Autodesk Inventor part; units mm, degrees
ref_plane "YZ Plane" through (0, 0, 0) normal (1, 0, 0) x (0, 1, 0)
ref_plane "XZ Plane" through (0, 0, 0) normal (0, 1, 0) x (-1, 0, 0)
ref_plane "XY Plane" through (0, 0, 0) normal (0, 0, 1) x (1, 0, 0)
ref_plane "作業平面1" through (0, 0, 0) normal (0, 0, 1) x (1, 0, 0)
sketch "スケッチ1" plane through (0, 0, 0) normal (0, 0, 1) x (1, 0, 0)
  circle A0 centre (16.5, -9.9) radius 0.8
  circle A1 centre (-18.5, 9.9) radius 0.8
  circle A2 centre (16.5, 9.9) radius 0.8
  circle A3 centre (-18.5, -9.9) radius 0.8
  arc A4 (-21.5, -7.9) -> (-23.5, -9.9) centre (-21.5, -9.9) ccw
  line L0 (-23.5, -9.9) -> (-23.5, -11.9)
  line L1 (-23.5, -11.9) -> (23.5, -11.9)
  line L2 (23.5, -11.9) -> (23.5, 11.9)
  line L3 (23.5, 11.9) -> (-23.5, 11.9)
  line L4 (-23.5, 11.9) -> (-23.5, 9.9)
  arc A5 (-23.5, 9.9) -> (-21.5, 7.9) centre (-21.5, 9.9) ccw
  line L5 (-21.5, 7.9) -> (21.5, 7.9)
  line L6 (21.5, 7.9) -> (21.5, -7.9)
  line L7 (21.5, -7.9) -> (-21.5, -7.9)
  line L8 (-21.5, 11.9) -> (-21.5, -11.9)
  point P0 (0, 0)
ref_plane "作業平面2" through (0, 0, 0) normal (0, 0, 1) x (1, 0, 0)
extrude "押し出し1" add sketch "スケッチ1" along normal blind 2 contours L8 L5 L6 L7 | L7 L6 L5 L8 L3 L2 L1
fillet "フィレット1" radius 2 4 edges at (23.5, 11.9, 1) (23.5, -11.9, 1) (-21.5, -11.9, 1) (-21.5, 11.9, 1)
sketch "スケッチ2" plane through (0, 0, 2) normal (0, 0, 1) x (1, 0, 0)
  line L0 (15.5, 8.9) -> (7, 8.9)
  line L1 (7, 8.9) -> (7, -8.9)
  line L2 (7, -8.9) -> (15.5, -8.9)
  line L3 (15.5, -8.9) -> (15.5, 8.9)
  circle A0 centre (16.5, 9.9) radius 0.8
  circle A1 centre (16.5, -9.9) radius 0.8
  point P0 (0, 0)
  dimension "d3" = 1
  dimension "d4" = 8.5
  dimension "d5" = 1
  dimension "d6" = 1
extrude "押し出し2" cut sketch "スケッチ2" against normal up to surface (2 mm away) contours L3 L2 L1 L0
properties part number "STlink_Top"
Part model, mm, in its own coordinate system. A direction names the side the tool comes from. Round coordinates to 2 decimals unless told otherwise and drop trailing zeros. Loops run counter-clockwise (first coordinate to the right, second up) from the corner with the lowest first, then second, coordinate; pieces in that order, holes last. Notation, with made-up numbers: (5, 51) -> (39, 51) arc R25 cw to (39, 73) -> close; hole circle Ø5 at (-15, 36.25). An arc over 180 degrees is marked (long way). Use CSV: the item, a comma, the result in double quotes. Start each with the question number.
1) Cut at A-A, the plane x = 16.5. Write the cut outline in (y, z), plus the area to 3 significant figures.
2) Cut at B-B, the plane y = 0. Write the cut outline in (x, z).
3) Wall check: L1, parallel to X at y = -10, z = 0.2; L2, parallel to Y at x = 16.5, z = 0.75; L3, parallel to Y at x = 14.5, z = 1.2. Give the ranges that are in metal, low to high. Write a range as [from, to].
4) Pull direction Z, two halves, no side cores. Call faces 1 (the cylindrical face through (15.87, -9.41, 0.99)), 2 (the flat face through (1, 0, 2)), 3 (the flat face through (1, 0, 0)): +Z half, -Z half, draft (parallel to the pull), parting line (faces both ways), or undercut.
5) Which spindle directions (+Z, -Z, +X, -X, +Y, -Y) get a long thin tool onto all of the face, cutting with end or side? Do faces 4 (the flat face through (7, 0, 1)), 5 (the flat face through (1, -11.9, 1)). Say none if no direction does.
6) Cut at C-C, the plane z = 1.2. Write the cut outline in (x, y), plus the area to 3 significant figures.
Determined:
1,outline,"(-11.9, 0) -> (-10.7, 0) -> (-10.7, 2) -> (-11.9, 2) -> close; (-9.1, 0) -> (9.1, 0) -> (9.1, 2) -> (-9.1, 2) -> close; (10.7, 0) -> (11.9, 0) -> (11.9, 2) -> (10.7, 2) -> close"
1,area,"41.2 mm2"
2,outline,"(-21.5, 0) -> (7, 0) -> (7, 2) -> (-21.5, 2) -> close; (15.5, 0) -> (23.5, 0) -> (23.5, 2) -> (15.5, 2) -> close"
3,L1,"x = [-21.5, -19.29], [-17.71, 15.71], [17.29, 23.5]"
3,L2,"y = [-11.9, -10.7], [-9.1, 9.1], [10.7, 11.9]"
3,L3,"y = [-11.9, -8.9], [8.9, 11.9]"
4,face 1,"draft"
4,face 2,"+Z half"
4,face 3,"-Z half"
5,face 4,"+Z, -Z"
5,face 5,"+Z, -Z, +X, -X, -Y"
6,outline,"(-21.5, -9.9) arc R2 ccw to (-19.5, -11.9) -> (21.5, -11.9) arc R2 ccw to (23.5, -9.9) -> (23.5, 9.9) arc R2 ccw to (21.5, 11.9) -> (-19.5, 11.9) arc R2 ccw to (-21.5, 9.9) -> close; hole circle Ø1.6 at (-18.5, -9.9); hole circle Ø1.6 at (-18.5, 9.9); hole (7, -8.9) -> (15.5, -8.9) -> (15.5, 8.9) -> (7, 8.9) -> close; hole circle Ø1.6 at (16.5, -9.9); hole circle Ø1.6 at (16.5, 9.9)"
6,area,"908 mm2"
